Geometry: final body of the model. Coordinates: model frame, mm. Face numbers are marked on the shaded views. A direction names the side the tool comes from. Round coordinates to 2 decimals unless told otherwise and drop trailing zeros. Order: outer loops, then holes, each group sorted by start corner. A loop starts at its lowest first (then second) coordinate and runs counter-clockwise, first axis right, second up. Notation, with made-up numbers: M 12,-3 L 48,-3 A13 cw 48,15 Z; hole C 59,17.5 d11. An arc over 180 degrees is marked long. Return JSON: item names as keys, results as strings. Group by question number.
Q1. Cut plane D-D on x = -26. Output: boundary loops of the cut face in (y, z).
Q2. Contact query for flat-ended pins moving along their axis: pin 1 (6 mm diameter, centred on x = -6.5, z = 19, fed in from +Y); pin 2 (3 mm diameter, centred on y = 13.5, z = -20, fed in from +X); pin 3 (8 mm diameter, centred on y = 8, z = 16.5, fed in from +X). Output: stop coordinate, or through.
Q3. Cut plane B-B on x = -1. Output: boundary loops of the cut face in (y, z).
Q4. Access query for the marked faces 1, 2 and 3. Directions: +Z, -Z, +X, -X, +Y, -Y. A direction counts if a zero-diameter tool reaches every point of the face in a straight line with its end or side. Return the directions, or none.
Q5. Cut plane C-C on z = 12.5. Output: boundary loops of the cut face in (x, y), and give its area (3 significant figures).
Q6. Ray query, probe 1 along Z at (x, y) = (30, 15.7); probe 2 along X at (y, z) = (15.7, -17.5); probe 3 along Z at (x, y) = (11, 9). Return the intervals inside material, ascending.
Q7. Cut plane A-A on y = 1.75. Output: boundary loops of the cut face in (x, z), and give its area (3 significant figures).
```python
from build123d import *

# Parameters (mm, degrees)
SKETCH1_W           = 80
SKETCH1_H           = 55
BOSS_EXTRUDE2_DEPTH = 20
FILLET1_R           = 10
SKETCH3_R           = 11
CUT_EXTRUDE2_DEPTH  = 6
SKETCH5_W           = 34
SKETCH5_H           = 18
CUT_EXTRUDE3_DEPTH  = 2
SKETCH6_R           = 10.5
BOSS_EXTRUDE3_DEPTH = 6
FILLET2_R           = 1
FILLET3_R           = 1
SKETCH7_W           = 34
SKETCH7_H           = 18
BOSS_EXTRUDE4_DEPTH = 2.5


with BuildPart() as part:
    # Sketch1 → Boss-Extrude2 (new body)
    with BuildSketch(Plane(origin=(0, 0, 0), x_dir=(1, 0, 0), z_dir=(0, 1, 0))):
        Rectangle(SKETCH1_W, SKETCH1_H)
    extrude(amount=BOSS_EXTRUDE2_DEPTH)

    # Fillet1
    fillet1_edges = [part.edges().sort_by_distance(p)[0] for p in [
        (40, 10, 27.5),
        (-40, 10, 27.5),
        (-40, 10, -27.5),
        (40, 10, -27.5),
    ]]
    fillet(fillet1_edges, radius=FILLET1_R)

    # Sketch3 → Cut-Extrude2 (cut)
    with BuildSketch(Plane(origin=(0, 20, 0), x_dir=(1, 0, 0), z_dir=(0, 1, 0))):
        with Locations((30, 17.5)):
            Circle(SKETCH3_R)
    extrude(amount=-CUT_EXTRUDE2_DEPTH, mode=Mode.SUBTRACT)

    # Sketch5 → Cut-Extrude3 (cut)
    with BuildSketch(Plane(origin=(0, 20, 0), x_dir=(1, 0, 0), z_dir=(0, 1, 0))):
        with Locations((-5, 13.5)):
            Rectangle(SKETCH5_W, SKETCH5_H)
    extrude(amount=-CUT_EXTRUDE3_DEPTH, mode=Mode.SUBTRACT)

    # Sketch6 → Boss-Extrude3 (add)
    with BuildSketch(Plane(origin=(0, 14, 0), x_dir=(1, 0, 0), z_dir=(0, 1, 0))):
        with Locations((30, 17.5)):
            Circle(SKETCH6_R)
    extrude(amount=BOSS_EXTRUDE3_DEPTH)

    # Fillet2
    fillet2_edges = [part.edges().sort_by_distance(p)[0] for p in [
        (-40, 20, 0),
        (40, 20, 2.291287847),
        (0, 20, 27.5),
        (-37.071067812, 20, 24.571067812),
        (37.071067812, 20, 24.571067812),
        (-37.071067812, 20, -24.571067812),
        (-2.291287847, 20, -27.5),
        (22.221825407, 20, -9.721825407),
    ]]
    fillet(fillet2_edges, radius=FILLET2_R)

    # Fillet3
    fillet3_edges = [part.edges().sort_by_distance(p)[0] for p in [
        (19.5, 20, -17.5),
    ]]
    fillet(fillet3_edges, radius=FILLET3_R)

    # Sketch7 → Boss-Extrude4 (add)
    with BuildSketch(Plane(origin=(0, 18, 0), x_dir=(1, 0, 0), z_dir=(0, 1, 0))):
        with Locations((-5, 13.5)):
            Rectangle(SKETCH7_W, SKETCH7_H)
    extrude(amount=BOSS_EXTRUDE4_DEPTH)


solid = part.part
```
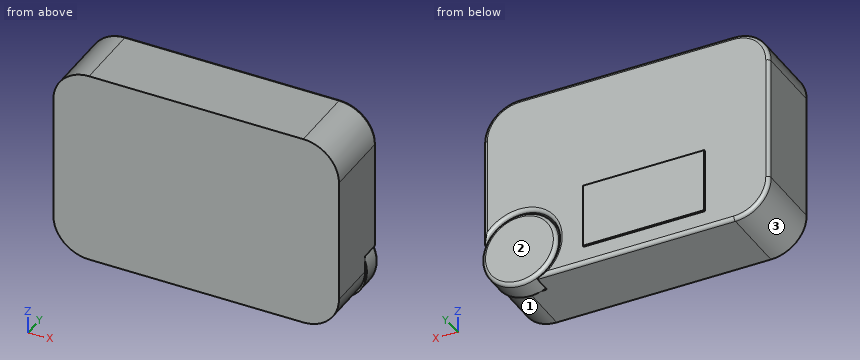
Result sheet:
{
 "1": {"outline": "M 0,-27.5 L 19,-27.5 A1 ccw 20,-26.5 L 20,26.5 A1 ccw 19,27.5 L 0,27.5 Z"},
 "2": {"pin 1": "stops at y = 20", "pin 2": "stops at x = 40.44", "pin 3": "stops at x = 40"},
 "3": {"outline": "M 0,-27.5 L 19,-27.5 A1 ccw 20,-26.5 L 20,-22.5 L 20.5,-22.5 L 20.5,-4.5 L 20,-4.5 L 20,26.5 A1 ccw 19,27.5 L 0,27.5 Z"},
 "4": {"face 1": "-Z, +X, -Y", "face 2": "+Z, -Z, +X, +Y", "face 3": "-Z, -X, +Y, -Y"},
 "5": {"outline": "M -40,0 L 40,0 L 40,19 A1 ccw 39,20 L -39,20 A1 ccw -40,19 Z", "area": "1,600 mm²"},
 "6": {"probe 1": "z = -28 to -7, -6.5 to 27.5", "probe 2": "x = -40 to 19, 19.5 to 40.5", "probe 3": "z = -27.5 to 27.5"},
 "7": {"outline": "M -40,-17.5 A10 ccw -30,-27.5 L 30,-27.5 A10 ccw 40,-17.5 L 40,17.5 A10 ccw 30,27.5 L -30,27.5 A10 ccw -40,17.5 Z", "area": "4,310 mm²"}
}
